```python
from build123d import *

# Parameters (mm, degrees)
F0_W     = 75
F0_H     = 8
F0_R     = 1.75
F0_W_2   = 56
F0_H_2   = 2
F1_DEPTH = 3
F3_DEPTH = 68
F4_W     = 5
F4_H     = 8
F5_DEPTH = 2
F6_SIZE  = 1.99999
F7_SIZE  = 0.99999
F8_SIZE  = 0.5


# Not quite as in the source:
# - a fillet or chamfer is up to 0.001 mm smaller than in the source, because OpenCascade refuses the exact size


with BuildPart() as f1:
    # F0 (on Top) → F1 (new body)
    with BuildSketch(Plane.XY):
        Rectangle(F0_W, F0_H)
        with Locations((-34.25, 0)):
            Circle(F0_R, mode=Mode.SUBTRACT)
        Rectangle(F0_W_2, F0_H_2, mode=Mode.SUBTRACT)
        with Locations((34.25, 0)):
            Circle(F0_R, mode=Mode.SUBTRACT)
    extrude(amount=F1_DEPTH)

    # F2 (on face) → F3 (join)
    with BuildSketch(Plane.XY.offset(3)):
        Polygon((-31, 4), (-31, -4), (-26, -4), (-26, -1), (-28, -1), (-28, 1), (28, 1), (28, -1), (26, -1), (26, -4), (31, -4), (31, 4), align=None)
    extrude(amount=F3_DEPTH)

    # F4 (on face) → F5 (join)
    with BuildSketch(Plane.XY.offset(71)):
        with Locations((-28.5, 0)):
            Rectangle(F4_W, F4_H)
        with Locations((28.5, 0)):
            Rectangle(F4_W, F4_H)
    extrude(amount=F5_DEPTH)

    # F6 (size 2 in the source; OpenCascade refuses exactly that, so slightly less here)
    f6_edges = [f1.edges().sort_by_distance(p)[0] for p in [
        (-26, 2.5, 71),
        (26, 2.5, 71),
    ]]
    chamfer(f6_edges, length=F6_SIZE)

    # F7 (size 1 in the source; OpenCascade refuses exactly that, so slightly less here)
    f7_edges = [f1.edges().sort_by_distance(p)[0] for p in [
        (-27, 1, 71),
        (27, 1, 71),
        (27, -1, 71),
        (-27, -1, 71),
    ]]
    chamfer(f7_edges, length=F7_SIZE)

    # F8
    f8_edges = [f1.edges().sort_by_distance(p)[0] for p in [
        (0, -1, 0),
        (0, 1, 0),
        (-28, 0, 0),
        (28, 0, 0),
    ]]
    chamfer(f8_edges, length=F8_SIZE)


solid = f1.part
```
Source: CAD feature listing. Evaluate the final solid. Frame: model axes, mm. A direction names the side the tool comes from. Round coordinates to 2 decimals unless told otherwise and drop trailing zeros. Loops run counter-clockwise (first coordinate to the right, second up) from the corner with the lowest first, then second, coordinate; pieces in that order, holes last. Notation, with made-up numbers: M 27.25,-39 L 79.25,-39 A23 ccw 79.25,-1 Z; hole C -18.75,41 d3. An arc over 180 degrees is marked long. Use a Markdown table: item, result. Add a question column.
1. Cut plane B-B, the plane z = 30.5. Output: boundary loops of the cut face in (x, y).
2. Cut plane D-D, the plane x = -34.25. Output: boundary loops of the cut face in (y, z), and give its area (3 significant figures).
3. Cut plane A-A, the plane x = 10. Output: boundary loops of the cut face in (y, z), and give its area (3 significant figures).
4. Cut plane C-C, the plane y = -3. Output: boundary loops of the cut face in (x, z).
5. Contact query for flat-ended pins moving along their axis: pin 1 (3 mm diameter, centred on x = 34, y = -1.5, fed in from +Z); pin 2 (1 mm diameter, centred on y = 0, z = 23.5, fed in from +X); pin 3 (1.5 mm diameter, centred on x = -7, y = 2.5, fed in from +Z); pin 4 (4 mm diameter, centred on x = 24.5, y = -1, fed in from -Z). Output: stop coordinate, or through.
6. Ray query, line 1 along X through (y, z) = (-1.25, 43); line 2 along X through (y, z) = (-0.5, 18); line 3 along Y through (x, z) = (26.5, 42). Return the intervals inside material, ascending. Write a range as [from, to].
7. Pull-direction query (X, two-part tool) for faces 6 (the flat face through (34, 2, 3)), 7 (the flat face through (37.5, 0, 1)), 8 (the flat face through (0, 3, 71)); classes: +X half, -X half, draft (parallel to the pull), parting line (faces both ways), or undercut.
8. Set-up query: faces 1 (the flat face through (-28, -4, 28)), 2 (the flat face through (-26, -2, 38)), 3 (the flat face through (-31, 0, 38)), 4 (the flat face through (28, 0, 35)), 5 (the flat face through (25, 2, 72)). Return all of +Z, -Z, +X, -X, +Y, -Y with unobstructed straight access to the full face (end or side cutting, diameter ignored); none if empty.
Solution:
| question | item | result |
|---|---|---|
| 1 | outline | M -31,-4 L -26,-4 L -26,-1 L -28,-1 L -28,1 L 28,1 L 28,-1 L 26,-1 L 26,-4 L 31,-4 L 31,4 L -31,4 Z |
| 2 | outline | M -4,0 L -1.75,0 L -1.75,3 L -4,3 Z; M 1.75,0 L 4,0 L 4,3 L 1.75,3 Z |
| 2 | area | 13.5 mm2 |
| 3 | outline | M -4,0 L -1.5,0 L -1,0.5 L -1,3 L -4,3 Z; M 1,0.5 L 1.5,0 L 4,0 L 4,71 L 1,71 Z |
| 3 | area | 222 mm2 |
| 4 | outline | M -37.5,0 L 37.5,0 L 37.5,3 L 31,3 L 31,73 L 26,73 L 26,3 L -26,3 L -26,73 L -31,73 L -31,3 L -37.5,3 Z |
| 5 | pin 1 | stops at z = 3 |
| 5 | pin 2 | stops at x = 31 |
| 5 | pin 3 | stops at z = 71 |
| 5 | pin 4 | stops at z = 0 |
| 6 | line 1 | x = [-31, -26], [26, 31] |
| 6 | line 2 | x = [-31, -28], [28, 31] |
| 6 | line 3 | y = [-4, -1], [1, 4] |
| 7 | face 6 | draft |
| 7 | face 7 | +X half |
| 7 | face 8 | undercut |
| 8 | face 1 | +Z, -Z, +X, -X, -Y |
| 8 | face 2 | +Z, -Y |
| 8 | face 3 | +Z, -X, +Y, -Y |
| 8 | face 4 | -Z |
| 8 | face 5 | +Z, +Y, -Y |
